```python
from build123d import *

# Parameters (mm, degrees)
F0_W     = 50.8
F0_H     = 25.4
F1_DEPTH = 38.1
F3_DEPTH = 12.7
F5_DEPTH = 12.7


with BuildPart() as f1:
    # F0 (on Front) → F1 (new body)
    with BuildSketch(Plane.XZ):
        with Locations((25.4, 12.7)):
            Rectangle(F0_W, F0_H)
    extrude(amount=F1_DEPTH)

    # F2 (on face) → F3 (cut)
    with BuildSketch(Plane.XY.offset(25.4)):
        Polygon((0, -38.1), (38.1, -38.1), (50.8, -19.05), (50.8, 0), (38.1, 0), (0, -31.75), align=None)
    extrude(amount=-F3_DEPTH, mode=Mode.SUBTRACT)

    # F4 (on face) → F5 (join)
    with BuildSketch(Plane.XY.offset(12.7)):
        Polygon((0, -38.1), (6.35, -38.1), (38.1, 0), (0, 0), align=None)
    extrude(amount=F5_DEPTH)


solid = f1.part
```
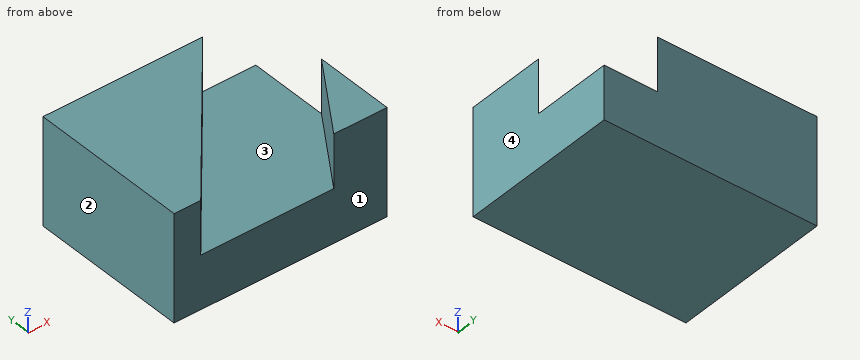
Model file for the job. Use its own axes, mm. Face numbers are marked on the shaded views. Coordinates: 2 decimals unless noted, no trailing zeros. Loops run counter-clockwise (first coordinate to the right, second up) from the corner with the lowest first, then second, coordinate; pieces in that order, holes last. Notation, with made-up numbers: (-6, 26) -> (3, 26) arc R30 ccw to (3, 50) -> close; hole circle Ø4 at (-21.5, -32.5). An arc over 180 degrees is marked (long way). Answer as a JSON object with one key per item and string values.
Q1. Cut at A-A (z = 17.25). List the corners of the cut face in (x, y), and give its area (3 significant figures).
Report:
{"outline": "(0, -38.1) -> (6.35, -38.1) -> (38.1, 0) -> (0, 0) -> close; (38.1, -38.1) -> (50.8, -38.1) -> (50.8, -19.05) -> close", "area": "968 mm2"}
Q2. Cut at C-C (x = 19.5). List the corners of the cut face in (y, z).
Report:
{"outline": "(-38.1, 0) -> (0, 0) -> (0, 25.4) -> (-22.32, 25.4) -> (-22.32, 12.7) -> (-38.1, 12.7) -> close"}
Q3. Cut at B-B (y = -30). List the corners of the cut face in (x, z).
Report:
{"outline": "(0, 0) -> (50.8, 0) -> (50.8, 25.4) -> (43.5, 25.4) -> (43.5, 12.7) -> (13.1, 12.7) -> (13.1, 25.4) -> (0, 25.4) -> close"}
Q4. Probe probe 1 along Z at (x, y) = (48.5, -13); probe 2 along X at (y, z) = (-20, 13.5); probe 3 along X at (y, z) = (-25.5, 17.5). List the from-to ranges inside material, lowest first.
Report:
{"probe 1": "z = 0 to 12.7", "probe 2": "x = 0 to 21.43, 50.17 to 50.8", "probe 3": "x = 0 to 16.85, 46.5 to 50.8"}
Q5. Flat gauge pin, fed straight in: P1, Ø5, axis at x = 18.5, z = 19, coming from the -Y side. Where does the tip first touch, or does it go through?
Report:
{"P1": "stops at y = -26.52"}
Q6. Cut at D-D (x = 12.5). List the corners of the cut face in (y, z), and give its area (3 significant figures).
Report:
{"outline": "(-38.1, 0) -> (0, 0) -> (0, 25.4) -> (-30.72, 25.4) -> (-30.72, 12.7) -> (-38.1, 12.7) -> close", "area": "874 mm2"}
Q7. Pull direction X, two halves, no side cores. Call the marked faces 1, 2, 3 and 4: released by +X, released by -X, zero draft, split by the parting line, or undercut.
Report:
{"face 1": "zero draft", "face 2": "released by -X", "face 3": "undercut", "face 4": "released by +X"}
